Autodesk Inventor part; units mm, degrees
ref_plane "YZ Plane" through (0, 0, 0) normal (1, 0, 0) x (0, 1, 0)
ref_plane "XZ Plane" through (0, 0, 0) normal (0, 1, 0) x (-1, 0, 0)
ref_plane "XY Plane" through (0, 0, 0) normal (0, 0, 1) x (1, 0, 0)
sketch "スケッチ1" plane through (0, 0, 0) normal (0, 0, 1) x (1, 0, 0)
  circle A0 centre (0, 0) radius 3
  circle A1 centre (0, 0) radius 1.5
  dimension "d0" = 6
  dimension "d1" = 3
extrude "押し出し1" add sketch "スケッチ1" along normal blind 20
fillet "フィレット1" radius 0.3 2 edges at (-3, 0, 20) (-3, 0, 0)
thread "ねじ1"
extrude "押し出し2" add sketch "スケッチ1" along normal blind 15 contours A1
extrude "押し出し3" cut sketch "スケッチ1" along normal blind 6 contours A1
thread "ねじ2"
properties part number "スペーサーM3L20アルミ" material "アルミニウム 2014-T4"
Here's how the part is built. I have some questions about the finished solid (model axes, mm). A direction names the side the tool comes from. Round coordinates to 2 decimals unless told otherwise and drop trailing zeros. Write each loop counter-clockwise with the first axis right and the second up, starting at its lowest first coordinate (ties: lowest second). Pieces come first, ordered by that corner, then holes. Notation, with made-up numbers: M 85.5,64 L 128.5,64 A24 cw 128.5,92 Z; hole C 33.5,40.5 d9. An arc over 180 degrees is marked long. Answer as CSV lines item,"result". Start each with the question number.
1. I'm going to push flat-ended pins straight in: pin 1 Ø3 at (x, y) = (2.5, 0) entering from -Z; pin 2 Ø2 at (y, z) = (-1.5, 8.5) entering from +X; pin 3 Ø0.9 at (x, y) = (-0.5, 0) entering from -Z; pin 4 Ø3 at (y, z) = (2, 17) entering from -X. Where does each tip first touch, or does it pass through?
2. Suppose I cut it at B-B on z = 6.75. Write out the boundary of the cut face in (x, y), then the cut area to 3 significant figures.
3. Thinking about a two-plate mould opening in Y: for faces 1 (the flat face through (0, 0, 6)), 2 (the cylindrical face through (-3, 0, 10)), 3 (the cylindrical face through (-1.5, -0.07, 2.96)), 4 (the flat face through (1.2, -1.2, 0)), which applies, released by +Y, released by -Y, zero draft, split by the parting line, or undercut?
4. Suppose I cut it at C-C on z = 17. Write out the boundary of the cut face in (x, y).
5. I need wall thicknesses on probe 1 along Y at (x, z) = (0, 17.3); probe 2 along Z at (x, y) = (1.25, 0); probe 3 along X at (y, z) = (-1.25, 18.25). Which ranges of each line are inside material? Lowest first, please.
6. Suppose I cut it at A-A on x = 0. Write out the boundary of the cut face in (y, z), then the cut area to 3 significant figures.
7. On a 3-axis mill with a long thin cutter (end or side, diameter ignored), from which of +Z, -Z, +X, -X, +Y, -Y can I reach the whole of each face in a straight line? I mean faces 5 (the flat face through (1.2, -1.2, 20)), 6 (the flat face through (0, 0, 15)). Say none if no direction works.
Check result:
1,pin 1,"stops at z = 0"
1,pin 2,"stops at x = 2.96"
1,pin 3,"stops at z = 6"
1,pin 4,"stops at x = -2.96"
2,outline,"C 0,0 d6"
2,area,"28.3 mm2"
3,face 1,"undercut"
3,face 2,"split by the parting line"
3,face 3,"undercut"
3,face 4,"zero draft"
4,outline,"C 0,0 d6; hole C 0,0 d3"
5,probe 1,"y = -3 to -1.5, 1.5 to 3"
5,probe 2,"z = 6 to 15"
5,probe 3,"x = -2.73 to -0.83, 0.83 to 2.73"
6,outline,"M -3,0.3 A0.3 ccw -2.7,0 L -1.5,0 L -1.5,6 L 1.5,6 L 1.5,0 L 2.7,0 A0.3 ccw 3,0.3 L 3,19.7 A0.3 ccw 2.7,20 L 1.5,20 L 1.5,15 L -1.5,15 L -1.5,20 L -2.7,20 A0.3 ccw -3,19.7 Z"
6,area,"86.9 mm2"
7,face 5,"+Z, +X, -X, +Y, -Y"
7,face 6,"+Z"
